Work out the finished part from the listing and answer in its coordinate system (mm). Face numbers are marked on the shaded views. A direction names the side the tool comes from. Round coordinates to 2 decimals unless told otherwise and drop trailing zeros. Write each loop counter-clockwise with the first axis right and the second up, starting at its lowest first coordinate (ties: lowest second). Pieces come first, ordered by that corner, then holes. Notation, with made-up numbers: (31.25, 32) - (59.25, 32) arc R29 ccw to (59.25, 54) - close; hole circle Ø1 at (5.25, -17.5). An arc over 180 degrees is marked (long way). Answer as a JSON object with one key per item and string values.
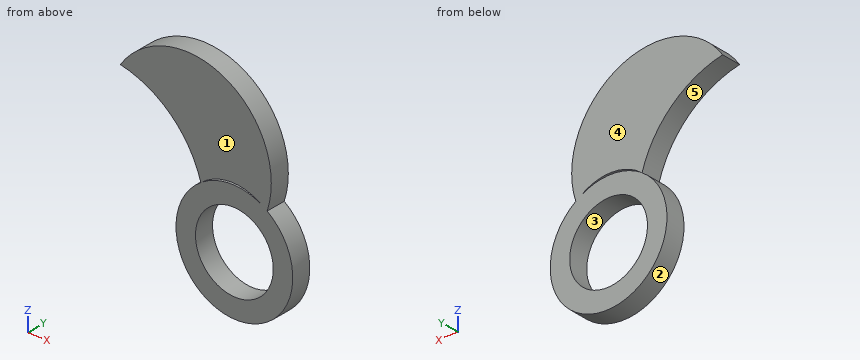
```python
from build123d import *

# Parameters (mm, degrees)
F0_R     = 7.62
F1_DEPTH = 1.27
F3_D     = 10.16
F5_DEPTH = 1.27


# Not quite as in the source:
# - a feature names something its author has since deleted; it is built from what else it names


with BuildPart() as f1:
    # F0 (on Front) → F1 (new body, symmetric)
    with BuildSketch(Plane.XZ):
        Circle(F0_R)
    extrude(amount=F1_DEPTH, both=True)

    # F3 (through all)
    with Locations(Plane.XZ.offset(1.27)):
        with Locations((0, 0)):
            Hole(F3_D / 2)

    # F4 (on Front) → F5 (join, symmetric)
    with BuildSketch(Plane.XZ):
        with BuildLine():
            ThreePointArc((-4.368594382, 6.2292921357), (-0.0581857965, 7.8272864293), (4.2522227889, 6.2292921357))
            ThreePointArc((4.2522227889, 6.2292921357), (-1.1998943931, 19.3169425848), (-14.8855810985, 15.6136797741))
            ThreePointArc((-14.8855810985, 15.6136797741), (-8.2843431722, 12.4262859834), (-4.368594382, 6.2292921357))
        make_face()
    extrude(amount=F5_DEPTH, both=True)


solid = f1.part
```
Item 1: A cutting plane is placed at C-C (x = -7). Write down the section's boundary in (y, z).
Results found:
{"outline": "(-1.27, -3.01) - (1.27, -3.01) - (1.27, 3.01) - (-1.27, 3.01) - close; (-1.27, 11.11) - (1.27, 11.11) - (1.27, 20.36) - (-1.27, 20.36) - close"}
Item 2: A cutting plane is placed at D-D (y = 0.35). Write down the section's boundary in (x, z).
Results found:
{"outline": "(-14.89, 15.61) arc R13.32 cw to (-4.37, 6.24) arc R7.62 ccw (long way) to (4.28, 6.31) arc R10.75 ccw to start; hole circle Ø10.16 at (0, 0); hole (-4.28, 6.31) arc R7.62 cw to (3.66, 6.69) arc R6.61 ccw to start"}
Item 3: Each of these flat-tipped pins is pushed along its axis until it touches: P1, Ø1.5, axis at x = 1.5, y = 1, coming from the +Z side; P2, Ø1, axis at x = -11, y = -1, coming from the -Z side. Where does it stop, or does it pass through?
Results found:
{"P1": "z = 18.09", "P2": "z = 14.03"}
Item 4: Determine the mould class of the marked faces 1, 2 and 3 for opening direction X: pulls with the +X half, pulls with the -X half, needs draft (parallel to the pull), parting line crosses it, or undercut.
Results found:
{"face 1": "needs draft", "face 2": "parting line crosses it", "face 3": "undercut"}
Item 5: Consider line 1 along Z through (x, y) = (0, 0.5); line 2 along Z through (x, y) = (-2.5, -0.3); line 3 along X through (y, z) = (0, 0.25). Determine where each line is inside the solid, lowest interval first.
Results found:
{"line 1": "-7.62 to -5.08, 5.08 to 7.62, 7.83 to 18.63", "line 2": "-7.2 to -4.42, 4.42 to 7.2, 7.36 to 19.85", "line 3": "-7.62 to -5.07, 5.07 to 7.62"}
Item 6: A cutting plane is placed at B-B (x = 0). Write down the section's boundary in (y, z).
Results found:
{"outline": "(-1.27, -7.62) - (1.27, -7.62) - (1.27, -5.08) - (-1.27, -5.08) - close; (-1.27, 5.08) - (1.27, 5.08) - (1.27, 7.62) - (-1.27, 7.62) - close; (-1.27, 7.83) - (1.27, 7.83) - (1.27, 18.63) - (-1.27, 18.63) - close"}
Item 7: For the marked faces 4 and 5, determine the directions among +Z, -Z, +X, -X, +Y, -Y from which every point of the face is accessible in a straight line to the end or side of a thin tool.
Results found:
{"face 4": "+Z, -Z, +X, -X, +Y", "face 5": "-X, +Y, -Y"}
Item 8: A cutting plane is placed at A-A (z = 0). Write down the section's boundary in (x, y).
Results found:
{"outline": "(-7.62, -1.27) - (-5.08, -1.27) - (-5.08, 1.27) - (-7.62, 1.27) - close; (5.08, -1.27) - (7.62, -1.27) - (7.62, 1.27) - (5.08, 1.27) - close"}
